Design review of the part built by this model. Coordinates are the model's own, in mm. A direction names the side the tool comes from. Give positions to 0.01 mm unless a question says otherwise; leave off trailing zeros. Write each loop counter-clockwise with the first axis right and the second up, starting at its lowest first coordinate (ties: lowest second). Pieces come first, ordered by that corner, then holes.
```python
from build123d import *

# Parameters (mm, degrees)
CROQUIS1_R              = 2
SALIENTE_EXTRUIR1_DEPTH = 10
SALIENTE_EXTRUIR2_START = 10
SALIENTE_EXTRUIR2_DEPTH = 10
CROQUIS3_R              = 0.75
CORTAR_EXTRUIR1_DEPTH   = 8


with BuildPart() as part:
    # Croquis1 → Saliente-Extruir1 (new, symmetric)
    with BuildSketch(Plane(origin=(0, 0, 0), x_dir=(1, 0, 0), z_dir=(0, 1, 0))):
        with Locations(Location((0, 0, 0), (0, 0, 270))):
            Circle(CROQUIS1_R)
    extrude(amount=SALIENTE_EXTRUIR1_DEPTH, both=True)

    # Croquis2 → Saliente-Extruir2 (add)
    with BuildSketch(Plane(origin=(0, 10, 0), x_dir=(1, 0, 0), z_dir=(0, 1, 0)).offset(SALIENTE_EXTRUIR2_START)):
        with BuildLine():
            Line((1.322875656, 1.5), (-1.322875656, 1.5))
            ThreePointArc((-1.322875656, 1.5), (-2, 0), (-1.322875656, -1.5))
            Line((-1.322875656, -1.5), (1.322875656, -1.5))
            ThreePointArc((1.322875656, -1.5), (2, 0), (1.322875656, 1.5))
        make_face()
    saliente_extruir2 = extrude(amount=-SALIENTE_EXTRUIR2_DEPTH)

    # Croquis3 → Cortar-Extruir1 (cut)
    with BuildSketch(Plane(origin=(0, 20, 0), x_dir=(1, 0, 0), z_dir=(0, 1, 0))):
        with Locations(Location((0, 0, 0), (0, 0, 270))):
            Circle(CROQUIS3_R)
    cortar_extruir1 = extrude(amount=-CORTAR_EXTRUIR1_DEPTH, mode=Mode.SUBTRACT)

    # Simetría1: Saliente-Extruir2, Cortar-Extruir1 across plane
    add(saliente_extruir2.mirror(Plane.ZX))
    add(cortar_extruir1.mirror(Plane.ZX), mode=Mode.SUBTRACT)


solid = part.part
```
(1) Consider section C-C, the plane y = 14. Give the boundary of the cut face in (x, z).
Resolved:
outline: (-1.32, -1.5) - (1.32, -1.5) arc R2 ccw to (1.32, 1.5) - (-1.32, 1.5) arc R2 ccw to start; hole circle Ø1.5 at (0, 0)
(2) Mouldability with a two-part tool opening along X and no side actions: class faces 4 (the face through (0, -20, 1)), 5 (the face through (0, 12, 0)) as pulls with the +X half, pulls with the -X half, needs draft (parallel to the pull), parting line crosses it, or undercut.
Resolved:
face 4: needs draft
face 5: undercut
(3) Consider section B-B, the plane x = 0. Give the boundary of the cut face in (y, z), then the cut area to 3 significant figures.
Resolved:
outline: (-20, -1.5) - (-10, -1.5) - (-10, -2) - (10, -2) - (10, -1.5) - (20, -1.5) - (20, -0.75) - (12, -0.75) - (12, 0.75) - (20, 0.75) - (20, 1.5) - (10, 1.5) - (10, 2) - (-10, 2) - (-10, 1.5) - (-20, 1.5) - (-20, 0.75) - (-12, 0.75) - (-12, -0.75) - (-20, -0.75) - close
area: 116 mm2
(4) Consider section A-A, the plane z = 0. Give the boundary of the cut face in (x, y).
Resolved:
outline: (-2, -20) - (-0.75, -20) - (-0.75, -12) - (0.75, -12) - (0.75, -20) - (2, -20) - (2, 20) - (0.75, 20) - (0.75, 12) - (-0.75, 12) - (-0.75, 20) - (-2, 20) - close
(5) Tool access review of faces 1 (the face through (0, 15, -1.5)), 2 (the face through (0.225, 16.056, 0.715)), 3 (the face through (0, 15, 1.5)): name each direction out of +Z, -Z, +X, -X, +Y, -Y from which nothing blocks a thin tool from reaching the whole face with its end or side.
Resolved:
face 1: -Z, +X, -X, +Y
face 2: +Y
face 3: +Z, +X, -X, +Y
(6) To check wall thickness, follow L1, parallel to X at y = -14.75, z = 0; L2, parallel to Z at x = -0.1, y = 15.5; L3, parallel to Y at x = -0.1, z = 1.6. State the ranges of each line that lie inside material, in increasing order.
Resolved:
L1: x = -2 to -0.75, 0.75 to 2
L2: z = -1.5 to -0.74, 0.74 to 1.5
L3: y = -10 to 10
(7) Clearance check with flat-ended pins moving along their axes: P1, Ø1.3, axis at x = 0.5, y = 15.5, coming from the +Z side; P2, Ø1.4, axis at x = 0, z = 0, coming from the +Y side; P3, Ø0.8, axis at x = 0, y = 15, coming from the -Z side. State where each tip first meets the part, or that it passes through.
Resolved:
P1: stops at z = 1.5
P2: stops at y = 12
P3: stops at z = -1.5
(8) Consider section D-D, the plane y = 9.5. Give the boundary of the cut face in (x, z), then the cut area to 3 significant figures.
Resolved:
outline: circle Ø4 at (0, 0)
area: 12.6 mm2
